```python
from build123d import *

# Parameters (mm, degrees)
F3_D     = 12
F3_DEPTH = 15
F3_TIP   = 3.6051637142
F6_D     = 12
F9_D     = 4.2
F9_DEPTH = 12
F9_START = 4.2023152
F9_TIP   = 1.2618073


with BuildPart() as f1:
    # F0 (on Top) → F1 (revolve)
    with BuildSketch(Plane.XY):
        with BuildLine():
            Line((0, 11), (0, 0))
            Line((0, 0), (61, 0))
            ThreePointArc((61, 0), (60.4959346906, 5.5901699437), (59, 11))
            Line((59, 11), (0, 11))
        make_face()
    revolve(axis=Axis((30.5, 0, 0), (1, 0, 0)))

    # F3
    with Locations(Plane(origin=(0, 0, 0), x_dir=(0, -1, 0), z_dir=(-1, 0, 0))):
        with Locations((0, 0)):
            Hole(F3_D / 2, depth=F3_DEPTH)
            with Locations((0, 0, -(F3_DEPTH + F3_TIP / 2))):  # 118° drill point
                Cone(0, F3_D / 2, F3_TIP, mode=Mode.SUBTRACT)

    # F6 (through all)
    with Locations(Plane(origin=(0, 15, 0), x_dir=(1, 0, 0), z_dir=(0, 1, 0))):
        with Locations((50, 0)):
            Hole(F6_D / 2)

    # F9
    # its depths count from where the whole tool has entered the part; down to there all is cleared
    with Locations(Plane.XY.offset(15).offset(-F9_START)):
        with Locations((5, 0), (47.5, 0)):
            Hole(F9_D / 2, depth=F9_DEPTH)
            with Locations((0, 0, -(F9_DEPTH + F9_TIP / 2))):  # 118° drill point
                Cone(0, F9_D / 2, F9_TIP, mode=Mode.SUBTRACT)


solid = f1.part
```
Could you check a few things on this model? Use its own coordinates, in mm. A direction names the side the tool comes from. Coordinates: 2 decimals unless noted, no trailing zeros. Write each loop counter-clockwise with the first axis right and the second up, starting at its lowest first coordinate (ties: lowest second). Pieces come first, ordered by that corner, then holes. Notation, with made-up numbers: (7, 71.25) -> (43, 71.25) arc R22 ccw to (43, 91.25) -> close; hole circle Ø8 at (80.5, 83). An arc over 180 degrees is marked (long way). Write item = value, one per line. Start each with the question number.
(1) I want a section at C-C (y = -9.25). Please give me the cut outline in (x, z).
(2) I want a section at D-D (x = 13). Please give me the cut outline in (y, z).
(3) I need wall thicknesses on line 1 (Z direction, x = 4, y = 0); line 2 (Y direction, x = 36, z = 0.25); line 3 (Y direction, x = 15.5, z = -3.5). Which ranges of each line are inside material? Lowest first, please. Write a range as [from, to].
(4) We'd pull the mould along Y, two halves only. Please class faces 1 (the face through (7.605, -1.301, -5.857)), 2 (the face through (0, 5, -5)), 3 (the face through (29.087, 5.076, -9.759)): released by +Y, released by -Y, zero draft, split by the parting line, or undercut.
(5) Which directions (+Z, -Z, +X, -X, +Y, -Y) give clear straight access to the entire face, cutting with the end or side of a thin tool? Please do faces 4 (the face through (54.42, -0.16, -4.06)), 5 (the face through (45.56, -0.8, 8.17)).
(6) I want a section at B-B (z = 9). Please give me the cut outline in (x, y).
(7) I want a section at A-A (x = 47.5). Please give me the cut outline in (y, z), plus the area to 3 significant figures.
(8) Will these pins go through, and if not, where does the flat tip stop? pin 1 (1.5 mm diameter, centred on x = 8, y = -2, fed in from -Z); pin 2 (12 mm diameter, centred on y = -1, z = 7.5, fed in from +X); pin 3 (4 mm diameter, centred on x = 5, y = 0, fed in from +Z).
Result set:
q1.outline = (0, -5.95) -> (49.25, -5.95) arc R6 cw to (49.25, 5.95) -> (0, 5.95) -> close; (50.75, -5.95) -> (59, -5.95) arc R29.85 ccw to (59, 5.95) -> (50.75, 5.95) arc R6 cw to start
q2.outline = circle Ø22 at (0, 0); hole circle Ø12 at (0, 0)
q3.line_1 = [-11, -6]
q3.line_2 = [-11, 11]
q3.line_3 = [-10.43, -3.8], [3.8, 10.43]
q4.face_1 = undercut
q4.face_2 = zero draft
q4.face_3 = split by the parting line
q5.face_4 = +Y, -Y
q5.face_5 = +Z
q6.outline = (0, -6.32) -> (59, -6.32) arc R29.93 ccw to (59, 6.32) -> (0, 6.32) -> close; hole circle Ø4.2 at (5, 0); hole circle Ø4.2 at (47.5, 0)
q7.outline = (-9.55, -5.45) arc R11 ccw to (9.55, -5.45) -> close; (-9.55, 5.45) -> (-2.1, 5.45) -> (-2.1, 10.8) arc R11 ccw to start; (2.1, 5.45) -> (9.55, 5.45) arc R11 ccw to (2.1, 10.8) -> close
q7.area = 127 mm2
q8.pin_1 = -10.93
q8.pin_2 = 60.96
q8.pin_3 = -5.66
